The listing builds one solid part. Answer for the finished solid, in the listing's coordinates (mm). A direction names the side the tool comes from. Round coordinates to 2 decimals unless told otherwise and drop trailing zeros. Order: outer loops, then holes, each group sorted by start corner. A loop starts at its lowest first (then second) coordinate and runs counter-clockwise, first axis right, second up. Notation, with made-up numbers: (54, 87) -> (81, 87) arc R13 cw to (81, 111) -> close; hole circle Ø1 at (82.5, -31.5). An arc over 180 degrees is marked (long way). Return JSON: item names as keys, results as strings. Group by question number.
(1) The part is cut by section C-C (x = 20.5). Determine the outline of the cut face in (y, z), plus the area to 3 significant figures.
(2) Determine the mould class of faces 1 (the face through (-1, -2, 25.5)), 2 (the face through (1, -1, 2)), 3 (the face through (97, 1, 0)) for opening direction Y: +Y half, -Y half, draft (parallel to the pull), parting line (faces both ways), or undercut.
(3) Each of these flat-tipped pins is pushed along its axis until it touches: pin 1 (0.5 mm diameter, centred on y = -0.5, z = 15.5, fed in from -X); pin 2 (1.2 mm diameter, centred on x = 55, y = -0.5, fed in from +Z). Where does it stop, or does it pass through?
(4) The part is cut by section B-B (y = -0.65). Determine the outline of the cut face in (x, z).
(5) Which of the six approach directions +Z, -Z, +X, -X, +Y, -Y give full straight-line access (tool end or side, diameter ignored) to faces 4 (the face through (-0.594, 0.493, -0.719)), 5 (the face through (166, -1, 1)), 6 (the face through (165.45, -0.76, 2.5))?
(6) The part is cut by section A-A (z = 13). Determine the outline of the cut face in (x, y).
(7) Consider line 1 (X direction, y = -0.1, z = 17); line 2 (X direction, y = -1.7, z = 18.75); line 3 (Z direction, x = 157.5, y = -1.3). Determine where each line is inside the solid, lowest interval first. Write a range as [from, to].
from build123d import *

# Parameters (mm, degrees)
F1_DEPTH = 1.5
F3_DEPTH = 1
F5_DEPTH = 1
F6_R     = 0.99999


# Not quite as in the source:
# - a fillet or chamfer is up to 0.001 mm smaller than in the source, because OpenCascade refuses the exact size
# - ends of sketch curves that miss each other by under 0.0002 mm in the source are joined


with BuildPart() as f1:
    # F0 (on Front) → F1 (new body)
    with BuildSketch(Plane.XZ):
        with BuildLine():
            Line((1.5, 25.5), (0, 25.5))
            Line((0, 25.5), (0, 5))
            ThreePointArc((0, 5), (1.4644660941, 1.4644660941), (5, 0))
            Line((5, 0), (163, 0))
            ThreePointArc((163, 0), (166.5355339059, 1.4644660941), (168, 5))
            Line((168, 5), (168, 25.5))
            Line((168, 25.5), (166.5, 25.5))
            Line((166.5, 25.5), (166.5, 5))
            ThreePointArc((166.5, 5), (165.4748737342, 2.5251262658), (163, 1.5))
            Line((163, 1.5), (5, 1.5))
            ThreePointArc((5, 1.5), (2.5251262658, 2.5251262658), (1.5, 5))
            Line((1.5, 5), (1.5, 25.5))
        make_face()
    extrude(amount=F1_DEPTH)

    # F2 (on face) → F3 (join)
    with BuildSketch(Plane.XZ.offset(1.5)):
        with BuildLine():
            Line((1.5, 5), (1.5, 25.5))
            Line((1.5, 25.5), (-3, 25.5))
            Line((-3, 25.5), (-3, 4.9999991791))
            ThreePointArc((-3, 4.9999991791), (-0.6568544899, -0.6568544899), (4.9999991791, -3))
            Line((4.9999991791, -3), (163, -3))
            ThreePointArc((163, -3), (168.6568542495, -0.6568542495), (171, 5))
            Line((171, 5), (171, 25.5))
            Line((171, 25.5), (166.5, 25.5))
            Line((166.5, 25.5), (166.5, 5))
            ThreePointArc((166.5, 5), (165.4748737342, 2.5251262658), (163, 1.5))
            Line((163, 1.5), (5, 1.5))
            ThreePointArc((5, 1.5), (2.5251257352, 2.5251263156), (1.5, 5))
        make_face()
    extrude(amount=F3_DEPTH)

    # F4 (on face) → F5 (join)
    with BuildSketch(Plane(origin=(0, 0, 0), x_dir=(-1, 0, 0), z_dir=(0, 1, 0))):
        with BuildLine():
            Line((-166.5, 5), (-166.5, 25.5))
            Line((-166.5, 25.5), (-171, 25.5))
            Line((-171, 25.5), (-171, 5))
            ThreePointArc((-171, 5), (-168.6568542495, -0.6568542495), (-163, -3))
            Line((-163, -3), (-5, -3))
            ThreePointArc((-5, -3), (0.6568542495, -0.6568542495), (3, 5))
            Line((3, 5), (3, 25.5))
            Line((3, 25.5), (-1.5, 25.5))
            Line((-1.5, 25.5), (-1.5, 5))
            ThreePointArc((-1.5, 5), (-2.5251262658, 2.5251262658), (-5, 1.5))
            Line((-5, 1.5), (-163, 1.5))
            ThreePointArc((-163, 1.5), (-165.4748737342, 2.5251262658), (-166.5, 5))
        make_face()
    extrude(amount=F5_DEPTH)

    # F6 (radius 1 in the source; OpenCascade refuses exactly that, so slightly less here)
    f6_edges = [f1.edges().sort_by_distance(p)[0] for p in [
        (165.474874, 1, 2.525126),
        (166.5, -2.5, 15.25),
    ]]
    fillet(f6_edges, radius=F6_R)


solid = f1.part
Answer below:
{
 "1": {"outline": "(-2.5, -3) -> (-1.5, -3) -> (-1.5, 0) -> (0, 0) -> (0, -3) -> (1, -3) -> (1, 0.5) arc R1 ccw to (0, 1.5) -> (-1.5, 1.5) arc R1 ccw to (-2.5, 0.5) -> close", "area": "10.8 mm²"},
 "2": {"face 1": "draft", "face 2": "undercut", "face 3": "+Y half"},
 "3": {"pin 1": "stops at x = 0", "pin 2": "stops at z = 1.5"},
 "4": {"outline": "(0, 5) arc R5 ccw to (5, 0) -> (163, 0) arc R5 ccw to (168, 5) -> (168, 25.5) -> (166.5, 25.5) -> (166.5, 5) arc R3.5 cw to (163, 1.5) -> (5, 1.5) arc R3.5 cw to (1.5, 5) -> (1.5, 25.5) -> (0, 25.5) -> close"},
 "5": {"face 4": "-Z, -X, +Y, -Y", "face 5": "-Z, +X", "face 6": "+Z, +Y, -Y"},
 "6": {"outline": "(-3, -2.5) -> (0.5, -2.5) arc R1 ccw to (1.5, -1.5) -> (1.5, 0) arc R1 ccw to (0.5, 1) -> (-3, 1) -> (-3, 0) -> (0, 0) -> (0, -1.5) -> (-3, -1.5) -> close; (166.5, -1.5) arc R1 ccw to (167.5, -2.5) -> (171, -2.5) -> (171, -1.5) -> (168, -1.5) -> (168, 0) -> (171, 0) -> (171, 1) -> (167.5, 1) arc R1 ccw to (166.5, 0) -> close"},
 "7": {"line 1": "x = [0, 1.5], [166.5, 168]", "line 2": "x = [-3, 1.48], [166.52, 171]", "line 3": "z = [0, 1.5]"}
}
